Geometry: final body of the model. Coordinates: model frame, mm. A direction names the side the tool comes from. Round coordinates to 2 decimals unless told otherwise and drop trailing zeros. Loops run counter-clockwise (first coordinate to the right, second up) from the corner with the lowest first, then second, coordinate; pieces in that order, holes last. Notation, with made-up numbers: (56.25, 40.25) - (97.25, 40.25) arc R20 ccw to (97.25, 78.25) - close; hole circle Ø9 at (35.5, -8.5). An arc over 180 degrees is marked (long way). Answer as CSV lines item,"result".
from build123d import *

# Parameters (mm, degrees)
EXTRUDE_2_DEPTH     = 9
SKETCH_4_R          = 2
SKETCH_4_R_2        = 3
CUT_EXTRUDE_1_DEPTH = 9
FILLET_1_R          = 1


with BuildPart() as part:
    # 草圖1 → 旋轉1 (revolve)
    with BuildSketch(Plane.XY, mode=Mode.PRIVATE) as revolve_1_sk:
        Polygon((25, 0), (0, 0), (0, 20), (11, 20), (11, 5), (25, 5), align=None)
    revolve(revolve_1_sk.sketch.rotate(Axis((0, 0, 0), (0, 1, 0)), 90), axis=Axis((0, 0, 0), (0, 1, 0)))

    # 草圖2 → 除料-旋轉1 (revolve, cut)
    with BuildSketch(Plane.XY, mode=Mode.PRIVATE) as cut_revolve_1_sk:
        Polygon((0, 20), (0, 0), (5, 0), (5, 17), (8, 17), (8, 20), align=None)
    revolve(cut_revolve_1_sk.sketch.rotate(Axis((0, 20, 0), (0, -1, 0)), 90), axis=Axis((0, 20, 0), (0, -1, 0)), mode=Mode.SUBTRACT)

    # 草圖3 → 填料-伸長2 (add)
    with BuildSketch(Plane(origin=(0, 0, 0), x_dir=(1, 0, 0), z_dir=(0, 1, 0))):
        with BuildLine():
            Line((-17, 5), (-9.797958971, 5))
            Line((-9.797958971, 5), (-9.797958971, -5))
            Line((-9.797958971, -5), (-17, -5))
            ThreePointArc((-17, -5), (-22, 0), (-17, 5))
        make_face()
        with BuildLine():
            Line((9.797958971, 5), (9.797958971, -5))
            Line((9.797958971, -5), (17, -5))
            ThreePointArc((17, -5), (22, 0), (17, 5))
            Line((17, 5), (9.797958971, 5))
        make_face()
    extrude(amount=EXTRUDE_2_DEPTH)

    # 草圖4 → 除料-伸長1 (cut)
    with BuildSketch(Plane(origin=(0, 0, 0), x_dir=(1, 0, 0), z_dir=(0, 1, 0))):
        with Locations(Location((-17.142374929, 0, 0), (0, 0, 270))):
            Circle(SKETCH_4_R)
        with Locations(Location((17, 0, 0), (0, 0, 270))):
            Circle(SKETCH_4_R)
        with Locations(Location((0, 18, 0), (0, 0, 90))):
            Circle(SKETCH_4_R_2)
        with Locations(Location((0, -18, 0), (0, 0, 90))):
            Circle(SKETCH_4_R_2)
    extrude(amount=CUT_EXTRUDE_1_DEPTH, mode=Mode.SUBTRACT)

    # 圓角1
    fillet_1_edges = [part.edges().sort_by_distance(p)[0] for p in [
        (0, 5, 25),
    ]]
    fillet(fillet_1_edges, radius=FILLET_1_R)


solid = part.part
(1) Draft query along X for faces 5 (the face through (4.213, 12.395, -10.161)), 6 (the face through (7.81, 18.52, -1.73)), 7 (the face through (14, 9, 0)). Return one class per face: pulls with the +X half, pulls with the -X half, needs draft (parallel to the pull), parting line crosses it, or undercut.
Findings below:
face 5,"parting line crosses it"
face 6,"undercut"
face 7,"needs draft"
(2) Pin query (flat end, axial travel): P1, Ø4, axis at x = -10, y = 8.5, coming from the -Z side; P2, Ø1, axis at y = 18, z = 2.5, coming from the -X side; P3, Ø3, axis at x = -13.5, z = 19.5, coming from the +Y side. Return the tip coordinate at first contact, or that it passes through.
Findings below:
P1,"z = -7.55"
P2,"x = -10.82"
P3,"y = 5"
(3) Material intervals for line 1 along X through (y, z) = (3.5, 0); line 2 along X through (y, z) = (7, 0); line 3 along Z through (x, y) = (-15, 6.25), sorted ascending.
Findings below:
line 1,"-25 to -19.14, -15.14 to -5, 5 to 15, 19 to 25"
line 2,"-22 to -19.14, -15.14 to -5, 5 to 15, 19 to 22"
line 3,"-5 to 5"
(4) Section B-B (y = 13.75). Output: boundary loops of the cut face in (x, z).
Findings below:
outline,"circle Ø22 at (0, 0); hole circle Ø10 at (0, 0)"
(5) Access query for faces 1 (the face through (-13, 7, 5)), 2 (the face through (22, 7, 0)), 3 (the face through (13, 7, -5)), 4 (the face through (13, 7, 5)). Directions: +Z, -Z, +X, -X, +Y, -Y. A direction counts if a zero-diameter tool reaches every point of the face in a straight line with its end or side. Return the directions, or none.
Findings below:
face 1,"+Z, -X, +Y"
face 2,"+X, +Y"
face 3,"-Z, +X, +Y"
face 4,"+Z, +X, +Y"
(6) Section A-A (z = 0). Give the number of separate pieces and of enclosed holes in the cut face, and give its area (3 significant figures).
Findings below:
separate pieces,"4"
enclosed holes,"0"
area,"378 mm2"
